Autodesk Inventor part; units mm, degrees
ref_plane "YZ Plane" through (0, 0, 0) normal (1, 0, 0) x (0, 1, 0)
ref_plane "XZ Plane" through (0, 0, 0) normal (0, 1, 0) x (-1, 0, 0)
ref_plane "XY Plane" through (0, 0, 0) normal (0, 0, 1) x (1, 0, 0)
sketch "Sketch1" plane through (0, 0, 0) normal (1, 0, 0) x (0, 1, 0)
  circle A0 centre (0, 0) radius 15
  dimension "d0" = 30
extrude "Extrusion1" add sketch "Sketch1" along normal blind 15
sketch "Sketch2" plane through (15, 0, 0) normal (1, 0, 0) x (0, 0, -1)
  circle A0 centre (0, 0) radius 8
  dimension "d3" = 16
extrude "Extrusion2" cut sketch "Sketch2" against normal blind 15
thread "Thread1"
sketch "Sketch3" plane through (15, 0, 0) normal (1, 0, 0) x (0, 0, -1)
  circle A0 centre (0, 0) radius 15
  line L0 (0, 15) -> (0, 13)
  line L1 (0, 13) -> (-2, 13)
  line L2 (-2, 13) -> (2, 13)
  line L3 (2, 13) -> (2, 17.4599)
  line L4 (2, 17.4599) -> (-2, 17.4599)
  line L5 (-2, 17.4599) -> (-2, 13)
  line L6 (-15, 0) -> (-13, 0)
  line L7 (-13, 0) -> (-13, -2)
  line L8 (-13, -2) -> (-13, 2)
  line L9 (-13, 2) -> (-17.4599, 2)
  line L10 (-17.4599, 2) -> (-17.4599, -2)
  line L11 (-17.4599, -2) -> (-13, -2)
  line L12 (0, -15) -> (0, -13)
  line L13 (0, -13) -> (2, -13)
  line L14 (2, -13) -> (-2, -13)
  line L15 (-2, -13) -> (-2, -17.4599)
  line L16 (-2, -17.4599) -> (2, -17.4599)
  line L17 (2, -17.4599) -> (2, -13)
  line L18 (15, 0) -> (13, 0)
  line L19 (13, 0) -> (13, 2)
  line L20 (13, 2) -> (13, -2)
  line L21 (13, -2) -> (17.4599, -2)
  line L22 (17.4599, -2) -> (17.4599, 2)
  line L23 (17.4599, 2) -> (13, 2)
  dimension "d8" = 2
  dimension "d9" = 2
  dimension "d10" = 4
  dimension "d13" = 360
extrude "Extrusion3" cut sketch "Sketch3" against normal blind 15 contours L18 L19 L23 A0 | A0 L23 L22 L21 | A0 L21 L20 L18 | L3 L2 L0 A0 | A0 L5 L4 L3 | L17 L16 L15 A0 | A0 L12 L13 L17 | L0 L1 L5 A0 | A0 L15 L14 L12 | L9 L8 L6 A0 | A0 L11 L10 L9 | A0 L6 L7 L11
properties part number "9. LockNutM16" material "Steel, Mild, Welded"
The model under review builds one solid part; all positions refer to its coordinate system, in mm. A direction names the side the tool comes from. Give positions to 0.01 mm unless a question says otherwise; leave off trailing zeros. Write each loop counter-clockwise with the first axis right and the second up, starting at its lowest first coordinate (ties: lowest second). Pieces come first, ordered by that corner, then holes.
1. Tool access review of faces 5 (the flat face through (8, -14, -2)), 6 (the flat face through (8, 14, 2)), 7 (the flat face through (8, -2, 14)): name each direction out of +Z, -Z, +X, -X, +Y, -Y from which nothing blocks a thin tool from reaching the whole face with its end or side.
2. For P1, Ø0.6, axis at x = 10, y = 14, coming from the +Z side; P2, Ø0.6, axis at x = 4.5, z = 14, coming from the -Y side; P3, Ø1.5, axis at x = 10.5, y = -14, coming from the -Z side; P4, Ø10, axis at y = -9.5, z = -4.5, coming from the -X side, all flat-tipped, find the tip position at first contact; note any pin that passes through.
3. Add section D-D, the plane z = -9. Write out the cut boundary in (x, y), plus the area to 3 significant figures.
4. Add section C-C, the plane x = 6.5. Write out the cut boundary in (y, z).
5. Add section A-A, the plane y = 0. Write out the cut boundary in (x, z), plus the area to 3 significant figures.
6. Wall thickness on L1, parallel to Y at x = 7.25, z = 0; L2, parallel to Z at x = 10.5, y = -6; L3, parallel to Y at x = 6.5, z = -1.5: over which ranges is each line inside the solid? List them lowest first.
7. Draft analysis for pull direction Y (two halves, no side actions). For faces 1 (the flat face through (8, 0, 13)), 2 (the flat face through (15, 6, -6)), 3 (the flat face through (8, 2, -14)), 4 (the flat face through (8, -13, 0)), state which applies: +Y half, -Y half, draft (parallel to the pull), parting line (faces both ways), or undercut.
Worked answers:
1. face 5: +X, -X, -Y
1. face 6: +X, -X, +Y
1. face 7: +Z, +X, -X
2. P1: stops at z = 6.11
2. P2: stops at y = -6.11
2. P3: stops at z = -7.03
2. P4: stops at x = 0
3. outline: (0, -12) - (15, -12) - (15, 12) - (0, 12) - close
3. area: 360 mm2
4. outline: (-14.87, -2) arc R15 ccw to (-2, -14.87) - (-2, -13) - (2, -13) - (2, -14.87) arc R15 ccw to (14.87, -2) - (13, -2) - (13, 2) - (14.87, 2) arc R15 ccw to (2, 14.87) - (2, 13) - (-2, 13) - (-2, 14.87) arc R15 ccw to (-14.87, 2) - (-13, 2) - (-13, -2) - close; hole circle Ø16 at (0, 0)
5. outline: (0, -13) - (15, -13) - (15, -8) - (0, -8) - close; (0, 8) - (15, 8) - (15, 13) - (0, 13) - close
5. area: 150 mm2
6. L1: y = -13 to -8, 8 to 13
6. L2: z = -13.75 to -5.29, 5.29 to 13.75
6. L3: y = -13 to -7.86, 7.86 to 13
7. face 1: undercut
7. face 2: draft
7. face 3: undercut
7. face 4: -Y half
